```python
from build123d import *

# Parameters (mm, degrees)
SKETCH_5_W          = 28
SKETCH_5_H          = 13
EXTRUDE_4_DEPTH     = 13.5
SKETCH_6_W          = 13.15
SKETCH_6_H          = 10.5
SKETCH_8_R          = 12
CUT_EXTRUDE_1_DEPTH = 13
SKETCH_9_W          = 28
SKETCH_9_H          = 13
EXTRUDE_5_DEPTH     = 1
SKETCH_11_W         = 13
SKETCH_11_H         = 14.5
EXTRUDE_6_DEPTH     = 1
FILLET_1_R          = 1
SKETCH_12_W         = 10
SKETCH_12_H         = 10
EXTRUDE_7_DEPTH     = 37.5
SKETCH_13_W         = 10
SKETCH_13_H         = 30
SKETCH_13_R         = 1
EXTRUDE_8_DEPTH     = 3.5
FILLET_2_R          = 2
FILLET_3_R          = 1


with BuildPart() as part:
    # 스케치5 → 보스-돌출4 (new body)
    with BuildSketch(Plane(origin=(0, 0, 0), x_dir=(1, 0, 0), z_dir=(0, 1, 0))):
        Rectangle(SKETCH_5_W, SKETCH_5_H)
    extrude(amount=EXTRUDE_4_DEPTH)

    # 컷-스윕1: sweep along a path in 스케치7
    with BuildLine(Plane.XY.offset(6.5)) as sweep_1_path:
        CenterArc((0, 0), 13.15, 0, 360)
    # 스케치6 → 컷-스윕1 (sweep, cut)
    with BuildSketch(Plane.XZ):
        with Locations((6.575, 0)):
            Rectangle(SKETCH_6_W, SKETCH_6_H)
    sweep(path=sweep_1_path.line, mode=Mode.SUBTRACT)

    # 스케치8 → 컷-돌출1 (cut)
    with BuildSketch(Plane.XY.offset(6.5)):
        Circle(SKETCH_8_R)
    extrude(amount=-CUT_EXTRUDE_1_DEPTH, mode=Mode.SUBTRACT)

    # 스케치9 → 보스-돌출5 (add)
    with BuildSketch(Plane(origin=(0, 13.5, 0), x_dir=(1, 0, 0), z_dir=(0, 1, 0))):
        Rectangle(SKETCH_9_W, SKETCH_9_H)
    extrude(amount=EXTRUDE_5_DEPTH)

    # 스케치11 → 보스-돌출6 (add)
    with BuildSketch(Plane(origin=(14, 0, 0), x_dir=(0, 0, -1), z_dir=(1, 0, 0))):
        with Locations((0, 7.25)):
            Rectangle(SKETCH_11_W, SKETCH_11_H)
    extrude(amount=EXTRUDE_6_DEPTH)

    # 필렛1
    fillet_1_edges = [part.edges().sort_by_distance(p)[0] for p in [
        (-14, 14.5, 0),
        (15, 14.5, 0),
    ]]
    fillet(fillet_1_edges, radius=FILLET_1_R)

    # 스케치12 → 보스-돌출7 (add)
    with BuildSketch(Plane.ZY.offset(14)):
        with Locations((0, 6.75)):
            Rectangle(SKETCH_12_W, SKETCH_12_H)
    extrude(amount=EXTRUDE_7_DEPTH)

    # 스케치13 → 보스-돌출8 (add)
    with BuildSketch(Plane.ZY.offset(51.5)):
        with Locations((0, 6.75)):
            Rectangle(SKETCH_13_W, SKETCH_13_H)
        with Locations((0, 16.75)):
            Circle(SKETCH_13_R, mode=Mode.SUBTRACT)
        with Locations((0, -3.25)):
            Circle(SKETCH_13_R, mode=Mode.SUBTRACT)
    extrude(amount=-EXTRUDE_8_DEPTH)

    # 필렛2
    # the kernel refuses this fillet: 2 mm, written as the material it adds along each edge
    with BuildSketch(Plane(origin=(-14, 11.75, 5), x_dir=(0, 0, 1), z_dir=(0, -1, 0)), Plane(origin=(-14, 1.75, -5), x_dir=(0, 0, -1), z_dir=(0, 1, 0))) as fillet_2_piece_1:
        with BuildLine():
            CenterArc((2, 1.936491673), FILLET_2_R, 180, 75.522487814)
            Line((0, 1.936491673), (-0.04, 1.936491673))
            Line((-0.04, 1.936491673), (-0.04, 0))
            Line((-0.04, 0), (0, -0.04))
            ThreePointArc((0, -0.04), (0.75, -0.04), (1.49, -0.038729833))
            Line((1.49, -0.038729833), (1.5, 0))
        make_face()
    extrude(amount=10)
    with BuildSketch(Plane(origin=(-14, 1.75, 5), x_dir=(0, -1, 0), z_dir=(0, 0, -1))) as fillet_2_piece_2:
        with BuildLine():
            CenterArc((2, 1.984313483), FILLET_2_R, 180, 82.819244219)
            Line((0, 1.984313483), (-0.04, 1.984313483))
            Line((-0.04, 1.984313483), (-0.04, 0))
            Line((-0.04, 0), (0, -0.04))
            ThreePointArc((0, -0.04), (0.875, -0.04), (1.745, -0.03968627))
            Line((1.745, -0.03968627), (1.75, 0))
        make_face()
    extrude(amount=10)
    with BuildSketch(Plane(origin=(-14, 11.75, 5), x_dir=(0, 0, 1), z_dir=(0, -1, 0))) as fillet_2_piece_3a_section:
        with BuildLine():
            CenterArc((2, 1.936491673), FILLET_2_R, 180, 75.522487814)
            Line((0, 1.936491673), (-0.04, 1.936491673))
            Line((-0.04, 1.936491673), (-0.04, 0))
            Line((-0.04, 0), (0, -0.04))
            ThreePointArc((0, -0.04), (0.75, -0.04), (1.49, -0.038729833))
            Line((1.49, -0.038729833), (1.5, 0))
        make_face()
    fillet_2_piece_3a = extrude(amount=14.841229183, mode=Mode.PRIVATE)
    fillet_2_piece_3a = split(fillet_2_piece_3a, bisect_by=Plane(origin=(-14.456288202, 0, 5.379183511), z_dir=(0, 1, 0)), keep=Keep.TOP, mode=Mode.PRIVATE)
    fillet_2_piece_3a = split(fillet_2_piece_3a, bisect_by=Plane(origin=(-14.456288202, 1.75, 5.379183511), z_dir=(0, -1, 0)), keep=Keep.TOP, mode=Mode.PRIVATE)
    with BuildSketch(Plane(origin=(-14, 1.75, 9.960783708), x_dir=(0, -1, 0), z_dir=(0, 0, -1))) as fillet_2_piece_3b_section:
        with BuildLine():
            CenterArc((2, 1.984313483), FILLET_2_R, 180, 82.819244219)
            Line((0, 1.984313483), (-0.04, 1.984313483))
            Line((-0.04, 1.984313483), (-0.04, 0))
            Line((-0.04, 0), (0, -0.04))
            ThreePointArc((0, -0.04), (0.875, -0.04), (1.745, -0.03968627))
            Line((1.745, -0.03968627), (1.75, 0))
        make_face()
    fillet_2_piece_3b = extrude(amount=14.960783708, mode=Mode.PRIVATE)
    fillet_2_piece_3b = split(fillet_2_piece_3b, bisect_by=Plane(origin=(-14.456897386, 1.324929313, 6.5), z_dir=(0, 0, -1)), keep=Keep.TOP, mode=Mode.PRIVATE)
    fillet_2_piece_3b = split(fillet_2_piece_3b, bisect_by=Plane(origin=(-14.456897386, 1.324929313, 5), z_dir=(0, 0, 1)), keep=Keep.TOP, mode=Mode.PRIVATE)
    fillet_2_piece_3 = fillet_2_piece_3a & fillet_2_piece_3b
    add(fillet_2_piece_3)
    with BuildSketch(Plane(origin=(-14, 1.75, 5), x_dir=(0, -1, 0), z_dir=(0, 0, -1))) as fillet_2_piece_4a_section:
        with BuildLine():
            CenterArc((2, 1.984313483), FILLET_2_R, 180, 82.819244219)
            Line((0, 1.984313483), (-0.04, 1.984313483))
            Line((-0.04, 1.984313483), (-0.04, 0))
            Line((-0.04, 0), (0, -0.04))
            ThreePointArc((0, -0.04), (0.875, -0.04), (1.745, -0.03968627))
            Line((1.745, -0.03968627), (1.75, 0))
        make_face()
    fillet_2_piece_4a = extrude(amount=14.960783708, mode=Mode.PRIVATE)
    fillet_2_piece_4a = split(fillet_2_piece_4a, bisect_by=Plane(origin=(-14.456897386, 1.324929313, -6.5), z_dir=(0, 0, 1)), keep=Keep.TOP, mode=Mode.PRIVATE)
    fillet_2_piece_4a = split(fillet_2_piece_4a, bisect_by=Plane(origin=(-14.456897386, 1.324929313, -5), z_dir=(0, 0, -1)), keep=Keep.TOP, mode=Mode.PRIVATE)
    with BuildSketch(Plane(origin=(-14, -3.091229183, -5), x_dir=(0, 0, -1), z_dir=(0, 1, 0))) as fillet_2_piece_4b_section:
        with BuildLine():
            CenterArc((2, 1.936491673), FILLET_2_R, 180, 75.522487814)
            Line((0, 1.936491673), (-0.04, 1.936491673))
            Line((-0.04, 1.936491673), (-0.04, 0))
            Line((-0.04, 0), (0, -0.04))
            ThreePointArc((0, -0.04), (0.75, -0.04), (1.49, -0.038729833))
            Line((1.49, -0.038729833), (1.5, 0))
        make_face()
    fillet_2_piece_4b = extrude(amount=14.841229183, mode=Mode.PRIVATE)
    fillet_2_piece_4b = split(fillet_2_piece_4b, bisect_by=Plane(origin=(-14.456288202, 0, -5.379183511), z_dir=(0, 1, 0)), keep=Keep.TOP, mode=Mode.PRIVATE)
    fillet_2_piece_4b = split(fillet_2_piece_4b, bisect_by=Plane(origin=(-14.456288202, 1.75, -5.379183511), z_dir=(0, -1, 0)), keep=Keep.TOP, mode=Mode.PRIVATE)
    fillet_2_piece_4 = fillet_2_piece_4a & fillet_2_piece_4b
    add(fillet_2_piece_4)

    # 필렛3
    # the kernel refuses this fillet: 1 mm, written as the material it adds along each edge
    with BuildSketch(Plane(origin=(-14, 11.75, 6.5), x_dir=(0, 1, 0), z_dir=(0, 0, -1))) as fillet_3_piece_1_section:
        with BuildLine():
            CenterArc((FILLET_3_R, -FILLET_3_R), FILLET_3_R, 90, 90)
            Line((0, -FILLET_3_R), (0, 0))
            Line((0, 0), (FILLET_3_R, 0))
        make_face()
    fillet_3_piece_1 = extrude(amount=13, mode=Mode.PRIVATE)
    fillet_3_piece_1 = fillet_3_piece_1 - Plane(origin=(-15.936491673, 11.983902991, -7), x_dir=(0, 0, -1), z_dir=(0, -1, 0)) * Cylinder(2, 30, mode=Mode.PRIVATE)
    fillet_3_piece_1 = fillet_3_piece_1 - Plane(origin=(-15.936491673, 11.983902991, 7), x_dir=(0, 0, 1), z_dir=(0, 1, 0)) * Cylinder(2, 30, mode=Mode.PRIVATE)
    add(fillet_3_piece_1)


solid = part.part
```
Input: part model. Units: mm. Frame: model coordinates. A direction names the side the tool comes from. Give positions to 0.01 mm unless a question says otherwise; leave off trailing zeros. Order: outer loops, then holes, each group sorted by start corner. A loop starts at its lowest first (then second) coordinate and runs counter-clockwise, first axis right, second up.
1. Draft query along Z for faces 1 (the face through (-49.774, 15.774, -0.217)), 2 (the face through (4, 12, 6.5)), 3 (the face through (-13.5, 0, -0.1)). Return one class per face: released by +Z, released by -Z, zero draft, split by the parting line, or undercut.
Computed:
face 1: undercut
face 2: released by +Z
face 3: zero draft
2. Cut plane C-C (y = -5). Return loops of the section in (x, z), and give its area (3 significant figures).
Computed:
outline: (-51.5, -5) - (-48, -5) - (-48, 5) - (-51.5, 5) - close
area: 35.0 mm2
3. Cut plane A-A (y = 16.75). Return loops of the section in (x, z), and give its area (3 significant figures).
Computed:
outline: (-51.5, -5) - (-48, -5) - (-48, -1) - (-51.5, -1) - close; (-51.5, 1) - (-48, 1) - (-48, 5) - (-51.5, 5) - close
area: 28.0 mm2
4. Set-up query: faces 4 (the face through (-48, 18, 0)), 5 (the face through (-51.5, 7, 0)), 6 (the face through (-38, 7, 5)), 7 (the face through (0, 14.5, 0)), 8 (the face through (-32, 1.75, 0)). Return all of +Z, -Z, +X, -X, +Y, -Y with unobstructed straight access to the full face (end or side cutting, diameter ignored); none if empty.
Computed:
face 4: +Z, -Z, +Y
face 5: +Z, -Z, -X, +Y, -Y
face 6: +Z, -X, +Y, -Y
face 7: +Z, -Z, +X, +Y
face 8: +Z, -Z, -Y
5. Pin query (flat end, axial travel): pin 1 Ø5 at (x, z) = (-24.5, 2.5) entering from +Y; pin 2 Ø10 at (x, y) = (-22.5, 13) entering from +Z; pin 3 Ø1.5 at (x, y) = (-37, 12) entering from -Z. Return the tip coordinate at first contact, or that it passes through.
Computed:
pin 1: stops at y = 11.75
pin 2: stops at z = 5
pin 3: stops at z = -5
6. Cut plane D-D (x = -39.5). Return loops of the section in (y, z).
Computed:
outline: (1.75, -5) - (11.75, -5) - (11.75, 5) - (1.75, 5) - close
7. Cut plane B-B (z = 0). Return loops of the section in (x, y).
Computed:
outline: (-51.5, -8.25) - (-48, -8.25) - (-48, -4.25) - (-51.5, -4.25) - close; (-51.5, -2.25) - (-48, -2.25) - (-48, 1.75) - (-15.98, 1.75) arc R2 cw to (-14, 0) - (-13.15, 0) arc R13.15 cw to (13.15, 0) - (15, 0) - (15, 13.5) arc R1 ccw to (14, 14.5) - (-13, 14.5) arc R1 ccw to (-14, 13.5) - (-14, 12.75) arc R1 cw to (-15, 11.75) - (-48, 11.75) - (-48, 15.75) - (-51.5, 15.75) - close; (-51.5, 17.75) - (-48, 17.75) - (-48, 21.75) - (-51.5, 21.75) - close
8. Line query: probe 1 along Y at (x, z) = (-49.85, 0); probe 2 along Y at (x, z) = (-32, 1.25); probe 3 along X at (y, z) = (1, 2.75). Output: solid intervals per line, ascending.
Computed:
probe 1: y = -8.25 to -4.25, -2.25 to 15.75, 17.75 to 21.75
probe 2: y = 1.75 to 11.75
probe 3: x = -51.5 to -48, -14.42 to -13.11, 13.11 to 15
